Read the model definition and answer for the solid it produces. Units are mm, in the model's axes. Coordinates: 2 decimals unless noted, no trailing zeros. Write each loop counter-clockwise with the first axis right and the second up, starting at its lowest first coordinate (ties: lowest second). Pieces come first, ordered by that corner, then holes. Notation, with made-up numbers: M -21,32 L -14,32 A25 ccw -14,71 Z; hole C 2.5,-30 d8. An arc over 180 degrees is marked long. Use a Markdown table: item, result. Add a question column.
Autodesk Inventor part; units mm, degrees
ref_plane "YZ Plane" through (0, 0, 0) normal (1, 0, 0) x (0, 1, 0)
ref_plane "XZ Plane" through (0, 0, 0) normal (0, 1, 0) x (-1, 0, 0)
ref_plane "XY Plane" through (0, 0, 0) normal (0, 0, 1) x (1, 0, 0)
sketch "Skizze1" plane through (0, 0, 0) normal (0, 1, 0) x (-1, 0, 0)
  line L0 (0, 0) -> (-708, 0)
  line L1 (-708, 0) -> (-708, 357)
  line L2 (-708, 357) -> (0, 357)
  line L3 (0, 357) -> (0, 0)
  line L4 (-354, 0) -> (-354, 357) construction
  line L5 (0, 178.5) -> (-708, 178.5) construction
  line L6 (-150, 0) -> (-150, 357) construction
  line L7 (-558, 0) -> (-558, 357) construction
  line L8 (-708, 67) -> (0, 67) construction
  line L9 (0, 71.4) -> (-708, 71.4) construction
  line L10 (-688, 337) -> (-688, 20) construction
  line L11 (-688, 20) -> (-20, 20) construction
  line L12 (-20, 20) -> (-20, 337) construction
  line L13 (-20, 337) -> (-688, 337) construction
  line L14 (-28, 19.5) -> (-12, 19.5) construction
  line L15 (-12, 19.5) -> (-12, 114.5) construction
  line L16 (-12, 114.5) -> (-28, 114.5) construction
  line L17 (-28, 114.5) -> (-28, 19.5) construction
  line L18 (-28, 19.5) -> (-12, 114.5) construction
  line L19 (-12, 19.5) -> (-28, 114.5) construction
  line L20 (-102.5, 345) -> (-197.5, 345) construction
  line L21 (-197.5, 345) -> (-197.5, 329) construction
  line L22 (-197.5, 329) -> (-102.5, 329) construction
  line L23 (-102.5, 329) -> (-102.5, 345) construction
  line L24 (-102.5, 345) -> (-197.5, 329) construction
  line L25 (-197.5, 345) -> (-102.5, 329) construction
  line L26 (-306.5, 345) -> (-401.5, 345) construction
  line L27 (-401.5, 345) -> (-401.5, 329) construction
  line L28 (-401.5, 329) -> (-306.5, 329) construction
  line L29 (-306.5, 329) -> (-306.5, 345) construction
  line L30 (-306.5, 345) -> (-401.5, 329) construction
  line L31 (-401.5, 345) -> (-306.5, 329) construction
  circle A0 centre (-20, 59.5) radius 3.25
  circle A1 centre (-20, 30) radius 4.5
  circle A2 centre (-20, 74.5) radius 3.25
  circle A3 centre (-20, 104) radius 4.5
  circle A4 centre (-142.5, 337) radius 3.25
  circle A5 centre (-113, 337) radius 4.5
  circle A6 centre (-317, 337) radius 4.5
  circle A7 centre (-346.5, 337) radius 3.25
  circle A8 centre (-157.5, 337) radius 3.25
  circle A9 centre (-187, 337) radius 4.5
  circle A10 centre (-391, 337) radius 4.5
  circle A11 centre (-361.5, 337) radius 3.25
  circle A12 centre (-688, 59.5) radius 3.25
  circle A13 centre (-688, 30) radius 4.5
  circle A14 centre (-688, 104) radius 4.5
  circle A15 centre (-688, 74.5) radius 3.25
  circle A16 centre (-565.5, 337) radius 3.25
  circle A17 centre (-595, 337) radius 4.5
  circle A18 centre (-550.5, 337) radius 3.25
  circle A19 centre (-521, 337) radius 4.5
  circle A20 centre (-150, 134) radius 3.25
  line L32 (-138.5, 124.5) -> (-161.5, 124.5) construction
  line L33 (-161.5, 124.5) -> (-161.5, 232.5) construction
  line L34 (-161.5, 232.5) -> (-138.5, 232.5) construction
  line L35 (-138.5, 232.5) -> (-138.5, 124.5) construction
  line L36 (-138.5, 124.5) -> (-161.5, 232.5) construction
  line L37 (-161.5, 124.5) -> (-138.5, 232.5) construction
  circle A21 centre (-150, 223) radius 3.25
  circle A22 centre (-558, 134) radius 3.25
  circle A23 centre (-558, 223) radius 3.25
  line L38 (-857.6188, 167) -> (175.5187, 167) construction
  line L39 (-857.6403, 142) -> (175.5402, 142) construction
  line L40 (-708, 317) -> (0, 317) construction
  line L41 (-668, 357) -> (-668, 0) construction
  line L42 (-708, 262) -> (-599.5, 262) construction
  line L43 (-613, 357) -> (-613, 217.4879) construction
  line L44 (-613, 357) -> (-708, 262)
  line L45 (-708, 3) -> (0, 3)
  point P0 (-20, 67)
  point P1 (-150, 337)
  point P2 (-354, 337)
  point P3 (-150, 178.5)
  dimension "d0" = 708
  dimension "d1" = 357
  dimension "d2" = 290
  dimension "d3" = 71.4
  dimension "d4" = 150
  dimension "d5" = 150
  dimension "d6" = 20
  dimension "d7" = 16
  dimension "d8" = 95
  dimension "d9" = 95
  dimension "d10" = 16
  dimension "d11" = 95
  dimension "d12" = 16
  dimension "d13" = 6.5
  dimension "d14" = 7.5
  dimension "d15" = 9
  dimension "d16" = 37
  dimension "d17" = 6.5
  dimension "d18" = 9
  dimension "d19" = 7.5
  dimension "d20" = 37
  dimension "d21" = 6.5
  dimension "d22" = 9
  dimension "d23" = 7.5
  dimension "d24" = 37
  dimension "d30" = 6.5
  dimension "d31" = 44.5
  dimension "d32" = 23
  dimension "d33" = 108
  dimension "d34" = 190
  dimension "d35" = 25
  dimension "d36" = 40
  dimension "d37" = 40
  dimension "d47" = 95
  dimension "d48" = 95
  dimension "d49" = 3
extrude "Ex1 mit Z-untermaß" add sketch "Skizze1" along normal blind 3 contours L45 L1 L44 L2 L3
chamfer "Fase1" distance 15 angle 45 3 edges at (0, 1.5, 357) (0, 1.5, 3) (708, 1.5, 3)
equation "\"d3\" = 0.2 * d1"
equation "\"d5\" = d4"
equation "\"d17\" = d13"
equation "\"d18\" = d15"
equation "\"d19\" = d14"
equation "\"d20\" = d16"
equation "\"d21\" = d13"
equation "\"d22\" = d15"
equation "\"d23\" = d14"
equation "\"d24\" = d16"
properties part number "enc-SidePanel 357x708"
Item 1: Find section B-B on z = 322.5. Give the vertices of the cut face in (x, y), then the cut area to 3 significant figures.
Item 2: Consider probe 1 along X at (y, z) = (1.55, 103); probe 2 along Z at (x, y) = (317, 1.45); probe 3 along Z at (x, y) = (361.5, 1.15). Determine where each line is inside the solid, lowest interval first.
Item 3: Find section A-A on y = 1.5. Count the separate pieces of the cut face and the enclosed holes in it, then the cut area to 3 significant figures.
Item 4: This flat-tipped pin is pushed along its axis until it touches: pin 1 (1 mm diameter, centred on y = 1, z = 291.5, fed in from +X). Where does it stop, or does it pass through?
Geometry says:
| question | item | result |
|---|---|---|
| 1 | outline | M 0,0 L 647.5,0 L 647.5,3 L 0,3 Z |
| 1 | area | 1,940 mm2 |
| 2 | probe 1 | x = 0 to 15.61, 24.39 to 683.61, 692.39 to 708 |
| 2 | probe 2 | z = 3 to 332.5, 341.5 to 357 |
| 2 | probe 3 | z = 3 to 333.75, 340.25 to 357 |
| 3 | separate pieces | 1 |
| 3 | enclosed holes | 24 |
| 3 | area | 245,000 mm2 |
| 4 | pin 1 | stops at x = 679 |
